Could you check a few things on this model? Use its own coordinates, in mm. A direction names the side the tool comes from. Round coordinates to 2 decimals unless told otherwise and drop trailing zeros. Loops run counter-clockwise (first coordinate to the right, second up) from the corner with the lowest first, then second, coordinate; pieces in that order, holes last. Notation, with made-up numbers: (37, 48) -> (74, 48) arc R19 ccw to (74, 66) -> close; hole circle Ø1 at (43.25, 50.5). An arc over 180 degrees is marked (long way). One line per item, written item: value.
```python
from build123d import *

# Parameters (mm, degrees)
SKETCH1_W           = 70
SKETCH1_H           = 60
ACRYLIC_BOARD_DEPTH = 3
SKETCH2_R           = 1.5
TO_CHASSIS_DEPTH    = 3
SKETCH3_R           = 1.5
SERVO_SCREW_DEPTH   = 3
SKETCH4_W           = 22
SKETCH4_H           = 41
SKETCH4_W_2         = 11
SKETCH4_H_2         = 26
SERVO_DEPTH         = 3
FILLET1_R           = 3


with BuildPart() as part:
    # Sketch1 → Acrylic Board (new body)
    with BuildSketch(Plane(origin=(0, 0, 0), x_dir=(1, 0, 0), z_dir=(0, 1, 0))):
        Rectangle(SKETCH1_W, SKETCH1_H)
    extrude(amount=ACRYLIC_BOARD_DEPTH)

    # Sketch2 → To Chassis (cut)
    with BuildSketch(Plane(origin=(0, 3, 0), x_dir=(1, 0, 0), z_dir=(0, 1, 0))):
        with Locations(Location((-30, 25, 0), (0, 0, 270))):
            Circle(SKETCH2_R)
        with Locations(Location((30, 25, 0), (0, 0, 270))):
            Circle(SKETCH2_R)
        with Locations(Location((30, 10, 0), (0, 0, 270))):
            Circle(SKETCH2_R)
        with Locations(Location((30, -5, 0), (0, 0, 270))):
            Circle(SKETCH2_R)
        with Locations(Location((30, -20, 0), (0, 0, 270))):
            Circle(SKETCH2_R)
        with Locations(Location((-30, 10, 0), (0, 0, 270))):
            Circle(SKETCH2_R)
        with Locations(Location((-30, -5, 0), (0, 0, 270))):
            Circle(SKETCH2_R)
        with Locations(Location((-30, -20, 0), (0, 0, 270))):
            Circle(SKETCH2_R)
    extrude(amount=-TO_CHASSIS_DEPTH, mode=Mode.SUBTRACT)

    # Sketch3 → Servo Screw (cut)
    with BuildSketch(Plane(origin=(0, 3, 0), x_dir=(1, 0, 0), z_dir=(0, 1, 0))):
        with Locations(Location((20, -25, 0), (0, 0, 270))):
            Circle(SKETCH3_R)
        with Locations(Location((15, -25, 0), (0, 0, 270))):
            Circle(SKETCH3_R)
        with Locations(Location((5, -25, 0), (0, 0, 270))):
            Circle(SKETCH3_R)
        with Locations(Location((10, -25, 0), (0, 0, 270))):
            Circle(SKETCH3_R)
        with Locations(Location((-5, -25, 0), (0, 0, 270))):
            Circle(SKETCH3_R)
        with Locations(Location((-10, -25, 0), (0, 0, 270))):
            Circle(SKETCH3_R)
        with Locations(Location((-15, -25, 0), (0, 0, 270))):
            Circle(SKETCH3_R)
        with Locations(Location((-15, 24, 0), (0, 0, 270))):
            Circle(SKETCH3_R)
        with Locations(Location((-10, 24, 0), (0, 0, 270))):
            Circle(SKETCH3_R)
        with Locations(Location((0, 24, 0), (0, 0, 270))):
            Circle(SKETCH3_R)
        with Locations(Location((5, 24, 0), (0, 0, 270))):
            Circle(SKETCH3_R)
        with Locations(Location((10, 24, 0), (0, 0, 270))):
            Circle(SKETCH3_R)
        with Locations(Location((15, 24, 0), (0, 0, 270))):
            Circle(SKETCH3_R)
        with Locations(Location((20, 24, 0), (0, 0, 270))):
            Circle(SKETCH3_R)
        with Locations(Location((0, -25, 0), (0, 0, 270))):
            Circle(SKETCH3_R)
        with Locations(Location((-5, 24, 0), (0, 0, 270))):
            Circle(SKETCH3_R)
    extrude(amount=-SERVO_SCREW_DEPTH, mode=Mode.SUBTRACT)

    # Sketch4 → Servo (cut)
    with BuildSketch(Plane(origin=(0, 3, 0), x_dir=(1, 0, 0), z_dir=(0, 1, 0))):
        with Locations((0, -0.5)):
            Rectangle(SKETCH4_W, SKETCH4_H)
        with Locations((-20.5, 10)):
            Rectangle(SKETCH4_W_2, SKETCH4_H_2)
    extrude(amount=-SERVO_DEPTH, mode=Mode.SUBTRACT)

    # Fillet1
    fillet1_edges = [part.edges().sort_by_distance(p)[0] for p in [
        (-35, 1.5, -30),
        (35, 1.5, -30),
        (35, 1.5, 30),
        (-35, 1.5, 30),
    ]]
    fillet(fillet1_edges, radius=FILLET1_R)


solid = part.part
```
(1) Imagine slicing it at D-D on x = 15. Write out the boundary of the cut face in (y, z), then the cut area to 3 significant figures.
Results below:
outline: (0, -30) -> (3, -30) -> (3, -25.5) -> (0, -25.5) -> close; (0, -22.5) -> (3, -22.5) -> (3, 23.5) -> (0, 23.5) -> close; (0, 26.5) -> (3, 26.5) -> (3, 30) -> (0, 30) -> close
area: 162 mm²
(2) Imagine slicing it at A-A on z = 5. Write out the boundary of the cut face in (x, y), then the cut area to 3 significant figures.
Results below:
outline: (-35, 0) -> (-31.5, 0) -> (-31.5, 3) -> (-35, 3) -> close; (-28.5, 0) -> (-11, 0) -> (-11, 3) -> (-28.5, 3) -> close; (11, 0) -> (28.5, 0) -> (28.5, 3) -> (11, 3) -> close; (31.5, 0) -> (35, 0) -> (35, 3) -> (31.5, 3) -> close
area: 126 mm²
(3) We'd pull the mould along Z, two halves only. Please class faces 1 (the face through (0, 2, 21)), 2 (the face through (-35, 1, 0)), 3 (the face through (-34.14, 1.52, 29.1)): +Z half, -Z half, draft (parallel to the pull), parting line (faces both ways), or undercut.
Results below:
face 1: undercut
face 2: draft
face 3: +Z half
(4) Imagine slicing it at C-C on x = 0. Write out the boundary of the cut face in (y, z).
Results below:
outline: (0, -30) -> (3, -30) -> (3, -25.5) -> (0, -25.5) -> close; (0, -22.5) -> (3, -22.5) -> (3, -20) -> (0, -20) -> close; (0, 21) -> (3, 21) -> (3, 23.5) -> (0, 23.5) -> close; (0, 26.5) -> (3, 26.5) -> (3, 30) -> (0, 30) -> close
(5) Imagine slicing it at B-B on x = -30. Write out the boundary of the cut face in (y, z).
Results below:
outline: (0, -30) -> (3, -30) -> (3, -26.5) -> (0, -26.5) -> close; (0, -23.5) -> (3, -23.5) -> (3, -11.5) -> (0, -11.5) -> close; (0, -8.5) -> (3, -8.5) -> (3, 3.5) -> (0, 3.5) -> close; (0, 6.5) -> (3, 6.5) -> (3, 18.5) -> (0, 18.5) -> close; (0, 21.5) -> (3, 21.5) -> (3, 30) -> (0, 30) -> close
(6) Please list where these lines run through material, in increasing order: L1, parallel to X at y = 1.95, z = -4; L2, parallel to Z at x = -17.5, y = 2.7; L3, parallel to X at y = 1.5, z = 12.5.
Results below:
L1: x = -35 to -26, -15 to -11, 11 to 35
L2: z = -30 to -23, 3 to 30
L3: x = -35 to -11, 11 to 35
(7) On a 3-axis mill with a long thin cutter (end or side, diameter ignored), from which of +Z, -Z, +X, -X, +Y, -Y can I reach the whole of each face in a straight line? I mean faces 4 (the face through (-11, 2, 1)), 5 (the face through (15, 0, 0)). Say none if no direction works.
Results below:
face 4: +Y, -Y
face 5: +Z, -Z, +X, -X, -Y
(8) For pin 1 Ø1.8 at (x, z) = (5, 25) entering from +Y, with a flat end and sliding along its axis, tell me the tip position at first contact or that it passes through.
Results below:
pin 1: passes through
